The model under review builds one solid part; all positions refer to its coordinate system, in mm. Face numbers are marked on the shaded views. A direction names the side the tool comes from. Coordinates: 2 decimals unless noted, no trailing zeros. Loops run counter-clockwise (first coordinate to the right, second up) from the corner with the lowest first, then second, coordinate; pieces in that order, holes last. Notation, with made-up numbers: (-20, 24.25) - (13, 24.25) arc R23 ccw to (13, 61.25) - close; hole circle Ø1 at (52.5, -24.75). An arc over 180 degrees is marked (long way). One line per item, written item: value. Start each with the question number.
1. Mouldability with a two-part tool opening along X and no side actions: class the marked faces 1, 2 and 3 as +X half, -X half, draft (parallel to the pull), parting line (faces both ways), or undercut.
2. We need section A-A, the plane x = 0. Give the boundary of the cut face in (y, z) (3 decimals), then the cut area to 3 significant figures.
3. For the marked faces 4, 5, 6 and 7, list the 3-axis set-ups (+Z, -Z, +X, -X, +Y, -Y) from which the entire face can be reached by the end or side of a thin tool; tool diameter is ignored.
4. To check wall thickness, follow line 1 (Y direction, x = 0, z = 2.35); line 2 (X direction, y = 4.25, z = 1.9); line 3 (Y direction, x = 12, z = 1.75). State the ranges of each line that lie inside material, in increasing order.
5. We need section B-B, the plane y = 0. Give the boundary of the cut face in (x, z) (3 decimals).
6. We need section C-C, the plane x = 6. Give the boundary of the cut face in (y, z) (3 decimals), then the cut area to 3 significant figures.
from build123d import *

# Parameters (mm, degrees)
SKETCH2_R           = 5
BOSS_EXTRUDE2_DEPTH = 3.175


with BuildPart() as part:
    # Sketch2 → Boss-Extrude2 (new body)
    with BuildSketch(Plane.XY):
        with BuildLine():
            ThreePointArc((9.456794765, 7.302125235), (10.51328966, 8.920913041), (10.82870315, 10.828049574))
            ThreePointArc((10.82870315, 10.828049574), (8.921045244, 10.513465667), (7.301533296, 9.457386704))
            ThreePointArc((7.301533296, 9.457386704), (5.308889045, 9.194845217), (4.539183834, 11.051485471))
            ThreePointArc((4.539183834, 11.051485471), (4.64471403, 12.981928422), (3.964051405, 14.791471183))
            ThreePointArc((3.964051405, 14.791471183), (2.469674584, 13.565372247), (1.59532555, 11.841424903))
            ThreePointArc((1.59532555, 11.841424903), (0.000409384, 10.617090374), (-1.594506782, 11.841424903))
            ThreePointArc((-1.594506782, 11.841424903), (-2.468043552, 13.565085875), (-3.961395494, 14.791451895))
            ThreePointArc((-3.961395494, 14.791451895), (-4.64300424, 12.982116437), (-4.538365066, 11.051485471))
            ThreePointArc((-4.538365066, 11.051485471), (-5.308070277, 9.194845217), (-7.300714528, 9.457386704))
            ThreePointArc((-7.300714528, 9.457386704), (-8.919846484, 10.513683908), (-10.827230806, 10.82870315))
            ThreePointArc((-10.827230806, 10.82870315), (-10.512252617, 8.921293027), (-9.455975997, 7.302125235))
            ThreePointArc((-9.455975997, 7.302125235), (-9.19343451, 5.309480984), (-11.050074764, 4.539775774))
            ThreePointArc((-11.050074764, 4.539775774), (-12.980517715, 4.64530597), (-14.790060475, 3.964643344))
            ThreePointArc((-14.790060475, 3.964643344), (-13.56396154, 2.470266524), (-11.840014195, 1.595917489))
            ThreePointArc((-11.840014195, 1.595917489), (-10.615679667, 0.001001323), (-11.840014195, -1.593914842))
            ThreePointArc((-11.840014195, -1.593914842), (-13.563675168, -2.467451613), (-14.790041187, -3.960803554))
            ThreePointArc((-14.790041187, -3.960803554), (-12.980705729, -4.6424123), (-11.050074764, -4.537773127))
            ThreePointArc((-11.050074764, -4.537773127), (-9.19343451, -5.307478337), (-9.455975997, -7.300122588))
            ThreePointArc((-9.455975997, -7.300122588), (-10.512273201, -8.919254544), (-10.827292443, -10.826638866))
            ThreePointArc((-10.827292443, -10.826638866), (-8.91988232, -10.511660678), (-7.300714528, -9.455384057))
            ThreePointArc((-7.300714528, -9.455384057), (-5.308070277, -9.19284257), (-4.538365066, -11.049482824))
            ThreePointArc((-4.538365066, -11.049482824), (-4.643895262, -12.979925775), (-3.963232637, -14.789468536))
            ThreePointArc((-3.963232637, -14.789468536), (-2.468855816, -13.5633696), (-1.594506782, -11.839422256))
            ThreePointArc((-1.594506782, -11.839422256), (0.000409384, -10.615087727), (1.59532555, -11.839422256))
            ThreePointArc((1.59532555, -11.839422256), (2.46886232, -13.563083228), (3.962214262, -14.789449248))
            ThreePointArc((3.962214262, -14.789449248), (4.643823008, -12.98011379), (4.539183834, -11.049482824))
            ThreePointArc((4.539183834, -11.049482824), (5.308889045, -9.19284257), (7.301533296, -9.455384057))
            ThreePointArc((7.301533296, -9.455384057), (8.920665252, -10.511681261), (10.828049574, -10.826700503))
            ThreePointArc((10.828049574, -10.826700503), (10.513071385, -8.91929038), (9.456794765, -7.300122588))
            ThreePointArc((9.456794765, -7.300122588), (9.194253278, -5.307478337), (11.050893532, -4.537773127))
            ThreePointArc((11.050893532, -4.537773127), (12.981336483, -4.643303323), (14.790879243, -3.962640697))
            ThreePointArc((14.790879243, -3.962640697), (13.564780308, -2.468263877), (11.840832964, -1.593914842))
            ThreePointArc((11.840832964, -1.593914842), (10.617899153, 0.000932392), (11.841424903, 1.59532555))
            ThreePointArc((11.841424903, 1.59532555), (13.565085875, 2.46886232), (14.791451895, 3.962214262))
            ThreePointArc((14.791451895, 3.962214262), (12.982116437, 4.643823008), (11.051485471, 4.539183834))
            ThreePointArc((11.051485471, 4.539183834), (9.193282623, 5.308357949), (9.456794765, 7.302125235))
        make_face()
        Circle(SKETCH2_R, mode=Mode.SUBTRACT)
    extrude(amount=BOSS_EXTRUDE2_DEPTH)


solid = part.part
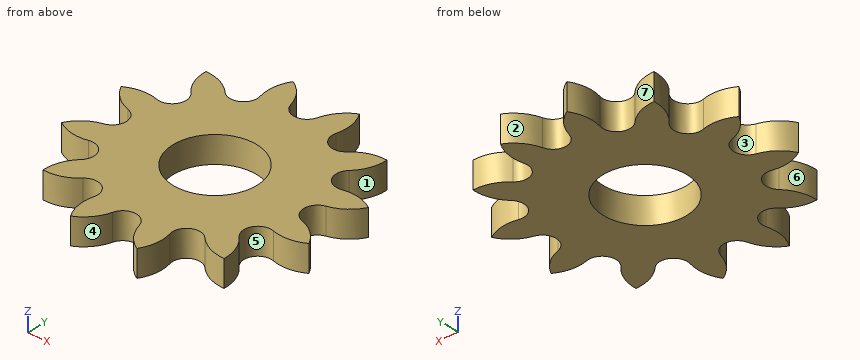
Findings below:
1. face 1: +X half
1. face 2: undercut
1. face 3: -X half
2. outline: (-10.615, 0) - (-5, 0) - (-5, 3.175) - (-10.615, 3.175) - close; (5, 0) - (10.617, 0) - (10.617, 3.175) - (5, 3.175) - close
2. area: 35.7 mm2
3. face 4: +Z, -Z, -Y
3. face 5: +Z, -Z
3. face 6: +Z, -Z, -X
3. face 7: +Z, -Z, +Y
4. line 1: -10.62 to -5, 5 to 10.62
4. line 2: -14.27 to -2.63, 2.63 to 14.27
4. line 3: -4.69 to -1.64, 1.64 to 4.69
5. outline: (-10.616, 0) - (-5, 0) - (-5, 3.175) - (-10.616, 3.175) - close; (5, 0) - (10.618, 0) - (10.618, 3.175) - (5, 3.175) - close
6. outline: (-8.977, 0) - (8.979, 0) - (8.979, 3.175) - (-8.977, 3.175) - close
6. area: 57.0 mm2
